For this review, use the dimensioned drawing (mm, ordinates from the lowest corner) and the shaded views. A direction names the side the tool comes from. Coordinates: 2 decimals unless noted, no trailing zeros. Loops run counter-clockwise (first coordinate to the right, second up) from the corner with the lowest first, then second, coordinate; pieces in that order, holes last. Notation, with made-up numbers: (51, 53) - (82, 53) arc R13 ccw to (82, 62) - close; hole circle Ø3 at (-27.5, 64). An arc over 180 degrees is marked (long way). Answer in a Markdown table with one row per item. Add a question column.
(1) For P1, Ø9, axis at x = 15.5, z = 38.5, coming from the -Y side; P2, Ø8, axis at x = 29, z = 20.5, coming from the +Y side; P3, Ø2, axis at y = 16.5, z = 34.5, coming from the -X side; P4, Ø19.5, axis at x = 22.5, y = 26, coming from the +Z side, all flat-tipped, find the tip position at first contact; note any pin that passes through.
(2) We need section A-A on y = 26. Write out the cut boundary in (x, z), plus the area to 3 significant figures.
(3) We need section B-B on x = 22.5. Write out the cut boundary in (y, z).
(4) Machinability: for the marked faces 1, 2, 3, 4 and 5, which of the approach directions +Z, -Z, +X, -X, +Y, -Y give a long, thin tool a straight path to every point of the face, cutting with its end or side? Answer none if there is none.
(5) For line 1 along Y through (x, z) = (22.5, 6); line 2 along X through (y, z) = (3, 35.5); line 3 along Z through (x, y) = (20.5, 36.5), list the stretches that pass through material, from the lowest coordinate up.
(6) Mouldability with a two-part tool opening along Y and no side actions: class the marked faces 6, 7, 8 and 9 as +Y half, -Y half, draft (parallel to the pull), parting line (faces both ways), or undercut.
(7) We need section C-C on z = 21.5. Write out the cut boundary in (x, y), plus the area to 3 significant figures.
(8) We need section D-D on y = 12. Write out the cut boundary in (x, z), plus the area to 3 significant figures.
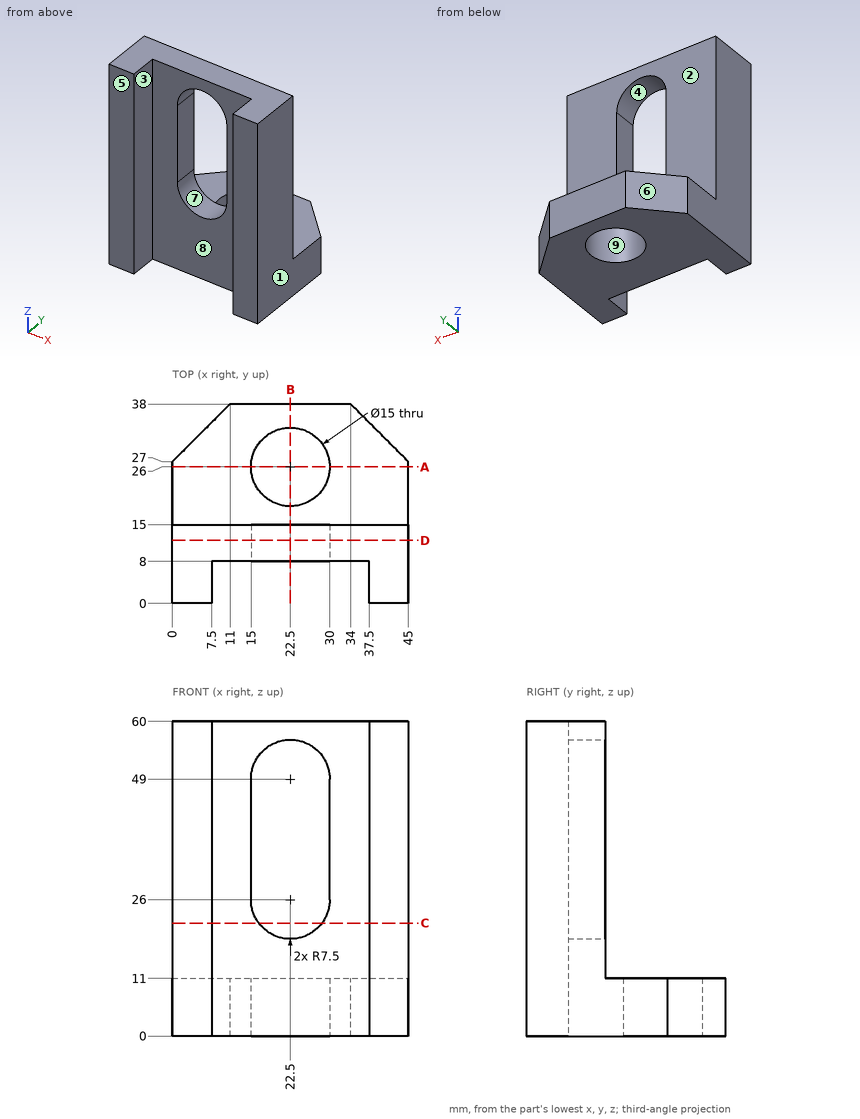
Outcome:
| question | item | result |
|---|---|---|
| 1 | P1 | y = 8 |
| 1 | P2 | y = 15 |
| 1 | P3 | through |
| 1 | P4 | z = 11 |
| 2 | outline | (0, 0) - (15, 0) - (15, 11) - (0, 11) - close; (30, 0) - (45, 0) - (45, 11) - (30, 11) - close |
| 2 | area | 330 mm² |
| 3 | outline | (8, 0) - (18.5, 0) - (18.5, 11) - (15, 11) - (15, 18.5) - (8, 18.5) - close; (8, 56.5) - (15, 56.5) - (15, 60) - (8, 60) - close; (33.5, 0) - (38, 0) - (38, 11) - (33.5, 11) - close |
| 4 | face 1 | +Z, -Z, +X, +Y, -Y |
| 4 | face 2 | +Z, +X, -X, +Y |
| 4 | face 3 | +Z, -Z, -Y |
| 4 | face 4 | +Y, -Y |
| 4 | face 5 | +Z, -Z, +X, -X, -Y |
| 5 | line 1 | 8 to 18.5, 33.5 to 38 |
| 5 | line 2 | 0 to 7.5, 37.5 to 45 |
| 5 | line 3 | 0 to 11 |
| 6 | face 6 | +Y half |
| 6 | face 7 | draft |
| 6 | face 8 | -Y half |
| 6 | face 9 | undercut |
| 7 | outline | (0, 0) - (7.5, 0) - (7.5, 8) - (16.5, 8) - (16.5, 15) - (0, 15) - close; (28.5, 8) - (37.5, 8) - (37.5, 0) - (45, 0) - (45, 15) - (28.5, 15) - close |
| 7 | area | 351 mm² |
| 8 | outline | (0, 0) - (45, 0) - (45, 60) - (0, 60) - close; hole (15, 26) arc R7.5 ccw to (30, 26) - (30, 49) arc R7.5 ccw to (15, 49) - close |
| 8 | area | 2,180 mm² |
